Source: CAD feature listing. Evaluate the final solid. Frame: model axes, mm. Give positions to 0.01 mm unless a question says otherwise; leave off trailing zeros. Write each loop counter-clockwise with the first axis right and the second up, starting at its lowest first coordinate (ties: lowest second). Pieces come first, ordered by that corner, then holes. Notation, with made-up numbers: (79.5, 52) - (95.5, 52) arc R20 ccw to (95.5, 85) - close; hole circle Ø5 at (42, -2). An arc over 180 degrees is marked (long way). Answer as a JSON object with one key per item and string values. Group by question number.
from build123d import *

# Parameters (mm, degrees)
SKETCH1_W               = 225.049134978
SKETCH1_H               = 177.4
BOSS_EXTRUDE1_DEPTH     = 1.5
CUT_EXTRUDE1_DEPTH      = 415.071536001
CUT_EXTRUDE1_DEPTH_BACK = 415.071536001
SKETCH2_W               = 37.712350792
SKETCH2_H               = 28.336351977


with BuildPart() as part:
    # Sketch1 → Boss-Extrude1 (new body)
    with BuildSketch(Plane.XY):
        with Locations((-223.710369918, -152.958961749)):
            Rectangle(SKETCH1_W, SKETCH1_H)
    extrude(amount=BOSS_EXTRUDE1_DEPTH)

    # Sketch2 → Cut-Extrude1 (cut, two sides: drawn at the far end of the back side and taken through both)
    with BuildSketch(Plane(origin=(0, 0, 0), x_dir=(-1, 0, 0), z_dir=(0, 0, -1)).offset(-CUT_EXTRUDE1_DEPTH_BACK)):
        with Locations((323.377350572, -181.028114896)):
            Rectangle(SKETCH2_W, SKETCH2_H)
    extrude(amount=CUT_EXTRUDE1_DEPTH + CUT_EXTRUDE1_DEPTH_BACK, mode=Mode.SUBTRACT)


solid = part.part
Q1. Ray query, probe 1 along Y at (x, z) = (-305.5, 0.45); probe 2 along X at (y, z) = (-169.5, 0.7). Return the intervals inside material, ascending. Write a range as [from, to].
Q2. Section A-A on x = -320.5. Return the cut outline in (y, z), then the cut area to 3 significant figures.
Q3. Section C-C on y = -170. Return the cut outline in (x, z).
Q4. Section B-B on z = 0.7. Return the cut outline in (x, y).
Taken from the geometry:
{
 "1": {"probe 1": "y = [-241.66, -195.2], [-166.86, -64.26]", "probe 2": "x = [-304.52, -111.19]"},
 "2": {"outline": "(-241.66, 0) - (-195.2, 0) - (-195.2, 1.5) - (-241.66, 1.5) - close; (-166.86, 0) - (-64.26, 0) - (-64.26, 1.5) - (-166.86, 1.5) - close", "area": "224 mm²"},
 "3": {"outline": "(-304.52, 0) - (-111.19, 0) - (-111.19, 1.5) - (-304.52, 1.5) - close"},
 "4": {"outline": "(-336.23, -241.66) - (-111.19, -241.66) - (-111.19, -64.26) - (-336.23, -64.26) - (-336.23, -166.86) - (-304.52, -166.86) - (-304.52, -195.2) - (-336.23, -195.2) - close"}
}
